Geometry: final body of the model. Coordinates: model frame, mm. A direction names the side the tool comes from. Give positions to 0.01 mm unless a question says otherwise; leave off trailing zeros. Order: outer loops, then holes, each group sorted by start corner. A loop starts at its lowest first (then second) coordinate and runs counter-clockwise, first axis right, second up. Notation, with made-up numbers: (-24, 79.5) -> (24, 79.5) arc R33 cw to (24, 111.5) -> close; hole circle Ø8 at (-25, 57). An arc over 180 degrees is marked (long way). Answer in a Markdown table with one row per item. Add a question column.
Q1. Cut plane C-C on z = 31.5. Return the cut outline in (x, y), and give its area (3 significant figures).
Q2. Pull-direction query (Y, two-part tool) for faces 1 (the face through (-48, -27, 20)), 2 (the face through (-19, 0, 3)), 3 (the face through (-82, -7, 3)); classes: +Y half, -Y half, draft (parallel to the pull), parting line (faces both ways), or undercut.
Q3. Set-up query: faces 4 (the face through (-69, -39, 11)), 5 (the face through (49.68, -60.08, 1.51)), 6 (the face through (26, -27, -7)). Return all of +Z, -Z, +X, -X, +Y, -Y with unobstructed straight access to the full face (end or side cutting, diameter ignored); none if empty.
Q4. Line query: line 1 along Y through (x, z) = (6.5, 13); line 2 along Y through (x, z) = (-63.5, -19); line 3 along X through (y, z) = (-61, -17). Output: solid intervals per line, ascending. Write a range as from..to.
Q5. Contact query for flat-ended pins moving along their axis: P1, Ø1, axis at y = -25, z = -14.5, coming from the -X side; P2, Ø4, axis at y = -55.5, z = 8, coming from the +X side; P3, Ø13.5, axis at y = -36.5, z = 20.5, coming from the +X side. Output: stop coordinate, or through.
Q6. Cut plane B-B on x = 11. Return the cut outline in (y, z).
Q7. Cut plane A-A on y = -46.5. Return the cut outline in (x, z).
Q8. Cut plane D-D on y = -68.5. Return the cut outline in (x, z).
from build123d import *

# Parameters (mm, degrees)
F1_DEPTH      = 84
F2_W          = 34
F2_H          = 25
F3_DEPTH      = 94.8
F3_DEPTH_BACK = 151.8
F4_W          = 48.559
F4_H          = 27
F4_W_2        = 16.441
F5_DEPTH      = 360.4


with BuildPart() as f1:
    # F0 (on Front) → F1 (new body)
    with BuildSketch(Plane.XZ):
        with BuildLine():
            Line((0, 45.618019), (-82, 45.618019))
            Line((-82, 45.618019), (-82, -41.381981))
            Line((-82, -41.381981), (-70, -41.381981))
            ThreePointArc((-70, -41.381981), (-32, -3.381981), (6, -41.381981))
            Line((6, -41.381981), (82, -41.381981))
            Line((82, -41.381981), (16.441, 45.618019))
            Line((16.441, 45.618019), (0, 45.618019))
        make_face()
    extrude(amount=F1_DEPTH)

    # F2 (on Top) → F3 (cut, two sides)
    with BuildSketch(Plane.XY) as f3_sk:
        with Locations((-65, -26.5)):
            Rectangle(F2_W, F2_H)
    extrude(amount=F3_DEPTH, mode=Mode.SUBTRACT)
    extrude(f3_sk.sketch, amount=-F3_DEPTH_BACK, mode=Mode.SUBTRACT)

    # F4 (on face) → F5 (cut)
    with BuildSketch(Plane.XY.offset(45.618019)):
        with Locations((40.7205, -40.5)):
            Rectangle(F4_W, F4_H)
        with Locations((8.2205, -40.5)):
            Rectangle(F4_W_2, F4_H)
    extrude(amount=-F5_DEPTH, mode=Mode.SUBTRACT)


solid = f1.part
Completed:
| question | item | result |
|---|---|---|
| 1 | outline | (-82, -84) -> (27.08, -84) -> (27.08, -54) -> (0, -54) -> (0, -27) -> (27.08, -27) -> (27.08, 0) -> (-82, 0) -> (-82, -14) -> (-48, -14) -> (-48, -39) -> (-82, -39) -> close |
| 1 | area | 7,580 mm² |
| 2 | face 1 | undercut |
| 2 | face 2 | +Y half |
| 2 | face 3 | draft |
| 3 | face 4 | +Z, -Z, -X |
| 3 | face 5 | +Z, +X, +Y, -Y |
| 3 | face 6 | +Z, -Z |
| 4 | line 1 | y = -84..-54, -27..0 |
| 4 | line 2 | y = -84..-39, -14..0 |
| 4 | line 3 | x = -82..-61.15, -2.85..63.63 |
| 5 | P1 | stops at x = -5.65 |
| 5 | P2 | stops at x = 46.3 |
| 5 | P3 | stops at x = 0 |
| 6 | outline | (-84, -41.38) -> (-54, -41.38) -> (-54, 45.62) -> (-84, 45.62) -> close; (-27, -41.38) -> (0, -41.38) -> (0, 45.62) -> (-27, 45.62) -> close |
| 7 | outline | (-82, -41.38) -> (-70, -41.38) arc R38 cw to (0, -20.89) -> (0, 45.62) -> (-82, 45.62) -> close; (65, -41.38) -> (82, -41.38) -> (65, -18.82) -> close |
| 8 | outline | (-82, -41.38) -> (-70, -41.38) arc R38 cw to (6, -41.38) -> (82, -41.38) -> (16.44, 45.62) -> (-82, 45.62) -> close |
